Solid Edge part; units mm, degrees
sketch "Sketch1" plane through (0, 0, 0) normal (0, -1, 0) x (1, 0, 0)
  line L0 (2.75, 5) -> (2.75, 0)
  line L1 (2.75, 0) -> (5, 0)
  line L2 (5, 0) -> (5, -8)
  line L3 (5, -8) -> (6, -8)
  arc A0 (6, -8) -> (7.4672, -6.8119) centre (6, -6.5) ccw
  line L4 (7.4672, -6.8119) -> (9.9779, 5)
  line L5 (9.9779, 5) -> (2.75, 5)
  dimension "D1" = 2.75
  dimension "D2" = 5
  dimension "D3" = 5
revolve "RevolvedProtrusion1" add sketch "Sketch1" angle 360 about axis through (0, 0, 0) along (0, 0, 1)
properties material "Bronze, 90%"
Model file for the job. Use its own axes, mm. A direction names the side the tool comes from. Give positions to 0.01 mm unless a question says otherwise; leave off trailing zeros. Loops run counter-clockwise (first coordinate to the right, second up) from the corner with the lowest first, then second, coordinate; pieces in that order, holes last.
Item 1: Drop flat-ended pins along their axis: P1, Ø1, axis at y = -4, z = -2.5, coming from the +X side; P2, Ø4.5, axis at x = 0, y = 0, coming from the -Z side; P3, Ø3, axis at x = 7.5, z = -3, coming from the +Y side; P4, Ø6, axis at x = 6.5, z = -0.5, coming from the -Y side. Give the stop position or say it passes through.
Check values:
P1: stops at x = 7.65
P2: passes through
P3: stops at y = 5.77
P4: stops at y = -8.25
Item 2: Slice it at D-D (z = 2.25). Write the cut outline in (x, y).
Check values:
outline: circle Ø18.79 at (0, 0); hole circle Ø5.5 at (0, 0)
Item 3: Drill centre lines: line 1 along X through (y, z) = (-3.5, -1.25); line 2 along Y through (x, z) = (0, -3.75); line 3 along Y through (x, z) = (-2, -0.75). Where is each one in solid material? Low to high.
Check values:
line 1: x = -7.91 to -3.57, 3.57 to 7.91
line 2: y = -8.12 to -5, 5 to 8.12
line 3: y = -8.52 to -4.58, 4.58 to 8.52
Item 4: Slice it at A-A (x = 0). Write the cut outline in (y, z).
Check values:
outline: (-9.98, 5) - (-7.47, -6.81) arc R1.5 ccw to (-6, -8) - (-5, -8) - (-5, 0) - (-2.75, 0) - (-2.75, 5) - close; (2.75, 0) - (5, 0) - (5, -8) - (6, -8) arc R1.5 ccw to (7.47, -6.81) - (9.98, 5) - (2.75, 5) - close
Item 5: Slice it at C-C (z = 0.25). Write the cut outline in (x, y), plus the area to 3 significant figures.
Check values:
outline: circle Ø17.94 at (0, 0); hole circle Ø5.5 at (0, 0)
area: 229 mm2
Item 6: Which spindle directions (+Z, -Z, +X, -X, +Y, -Y) get a long thin tool onto all of the face, cutting with end or side? Do faces 1 (the face through (-4, 4, -8)), 2 (the face through (-1.08, 4.88, -4.06)). Say none if no direction does.
Check values:
face 1: -Z, +X, -X, +Y, -Y
face 2: -Z
